Work out the finished part from the listing and answer in its coordinate system (mm). A direction names the side the tool comes from. Coordinates: 2 decimals unless noted, no trailing zeros. Order: outer loops, then holes, each group sorted by start corner. A loop starts at its lowest first (then second) coordinate and runs counter-clockwise, first axis right, second up. Notation, with made-up numbers: M 52.5,-28 L 75.5,-28 A21 cw 75.5,-5 Z; hole C 80.25,-0.75 d7. An arc over 180 degrees is marked long. Write item = value, one per line. Start each with the question number.
Q1. Straight lines are drawn through the part: line 1 along Z through (x, y) = (-33, 2.75); line 2 along Y through (x, z) = (-1, -11); line 3 along Y through (x, z) = (-32, -25). For each, find the intervals that lie inside material, in ascending order.
Q2. Find section D-D on x = 28. Give the vertices of the cut face in (y, z).
Q3. Each of these flat-tipped pins is pushed along its axis until it touches: P1, Ø17.5, axis at x = 41.5, z = -12.5, coming from the -Y side; P2, Ø9, axis at x = 5.5, z = -8, coming from the -Y side; P3, Ø4, axis at x = -9, y = 10, coming from the -Z side; P4, Ø1.5, axis at y = 9.5, z = -26.5, coming from the -X side. Where does it stop, or does it pass through?
Q4. A tool of negligible diameter and unlimited length cuts with its end or side. For faces 1 (the flat face through (-31, -2, -25.4)), 2 (the flat face through (-44, 7.585, -13)), 3 (the cylindrical face through (-30.669, 6.258, -27.904)), from which of +Z, -Z, +X, -X, +Y, -Y can it reach the whole face along a straight path? Write none if from no direction.
Q5. Find section B-B on x = -33. Give the vertices of the cut face in (y, z).
Q6. Find section A-A on y = -7.25. Give the vertices of the cut face in (x, z), and give its area (3 significant figures).
Q7. Determine the mould class of faces 4 (the flat face through (32.122, 13.382, -12.522)), 5 (the flat face through (45, 0, -13)), 6 (the flat face through (0, 8, -25.4)) for opening direction X: released by +X, released by -X, zero draft, split by the parting line, or undercut.
Q8. Find section C-C on z = -19. Give the vertices of the cut face in (x, y).
```python
from build123d import *

# Parameters (mm, degrees)
F1_DEPTH = 25.4
F2_R     = 6.666514
F2_R_2   = 8.083865
F3_DEPTH = 25.4
F5_DEPTH = 30.48


with BuildPart() as f1:
    # F0 (on Top) → F1 (new body)
    with BuildSketch(Plane.XY):
        with BuildLine():
            Line((-51.390246, 7.585276), (-51.390246, 0))
            Line((-51.390246, 0), (-36.978222, 0))
            ThreePointArc((-36.978222, 0), (-30.530737, 4.941209), (-24.083251, 0))
            Line((-24.083251, 0), (21.807669, 0))
            ThreePointArc((21.807669, 0), (29.582576, 5.313651), (37.357483, 0))
            Line((37.357483, 0), (53.286567, 0))
            Line((53.286567, 0), (53.286567, 7.585276))
            Line((53.286567, 7.585276), (37.357483, 7.585276))
            Line((37.357483, 7.585276), (26.7381, 19.342454))
            Line((26.7381, 19.342454), (-24.083251, 19.342454))
            Line((-24.083251, 19.342454), (-36.978222, 7.585276))
            Line((-36.978222, 7.585276), (-51.390246, 7.585276))
        make_face()
    extrude(amount=-F1_DEPTH)

    # F2 (on Top) → F3 (join)
    with BuildSketch(Plane.XY):
        with Locations((-30.776636, -2.161567)):
            Circle(F2_R)
        with Locations((29.519783, -2.172714)):
            Circle(F2_R_2)
    extrude(amount=-F3_DEPTH)

    # F4 (on Top) → F5 (join)
    with BuildSketch(Plane.XY):
        with BuildLine():
            Line((-25.728483, 0), (-23.92667, 0))
            ThreePointArc((-23.92667, 0), (-30.812173, 6.259093), (-37.697677, 0))
            Line((-37.697677, 0), (-36.024563, 0))
            ThreePointArc((-36.024563, 0), (-30.876523, 4.711429), (-25.728483, 0))
        make_face()
        with BuildLine():
            Line((34.646899, 0), (37.195049, 0))
            ThreePointArc((37.195049, 0), (29.186578, 6.065914), (21.178108, 0))
            Line((21.178108, 0), (23.180226, 0))
            ThreePointArc((23.180226, 0), (28.913562, 4.008779), (34.646899, 0))
        make_face()
    extrude(amount=-F5_DEPTH)


solid = f1.part
```
Findings below:
q1.line_1 = -25.4 to 0
q1.line_2 = 0 to 19.34
q1.line_3 = -8.71 to 4.39, 4.59 to 12.12
q2.outline = M -10.11,-25.4 L 3.94,-25.4 L 3.94,-30.48 L 5.98,-30.48 L 5.98,-25.4 L 17.95,-25.4 L 17.95,0 L -10.11,0 Z
q3.P1 = -9.58
q3.P2 = 0
q3.P3 = -25.4
q3.P4 = through
q4.face_1 = -Z, -Y
q4.face_2 = +Z, -Z, -X, +Y
q4.face_3 = -Z, +Y
q5.outline = M -8.45,-25.4 L 4.12,-25.4 L 4.12,0 L -8.45,0 Z; M 4.26,-30.48 L 5.9,-30.48 L 5.9,-25.4 L 11.21,-25.4 L 11.21,0 L 4.26,0 Z
q6.outline = M -35.08,-25.4 L -26.47,-25.4 L -26.47,0 L -35.08,0 Z; M 23.23,-25.4 L 35.81,-25.4 L 35.81,0 L 23.23,0 Z
q6.area = 538 mm^2
q7.face_4 = released by +X
q7.face_5 = zero draft
q7.face_6 = undercut
q8.outline = M -51.39,0 L -37.08,0 A6.67 ccw long -24.47,0 L 21.73,0 A8.08 ccw long 37.17,0.45 A8.34 cw 37.36,0 L 53.29,0 L 53.29,7.59 L 37.36,7.59 L 26.74,19.34 L -24.08,19.34 L -36.98,7.59 L -51.39,7.59 Z; hole M -33.93,3.71 A6.67 cw -28.33,4.04 A5.17 ccw Z
